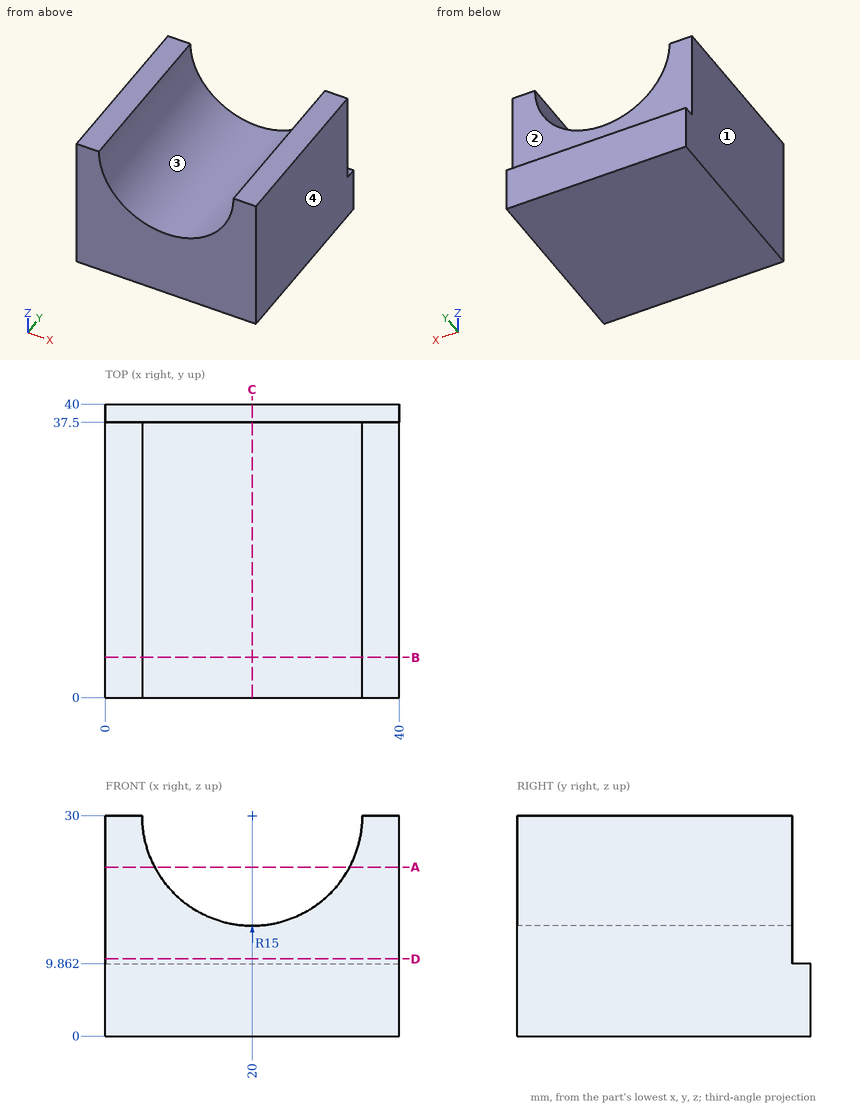
Can you work these out from the drawing? Everything is in mm from the part's minimum corner. Give positions to 0.01 mm unless a question says otherwise; leave off trailing zeros. Order: outer loops, then holes, each group sorted by start corner. A loop starts at its lowest first (then second) coordinate and runs counter-clockwise, first axis right, second up. Notation, with made-up numbers: M -38,-1 L 21,-1 A27 ccw 21,22 Z; hole C 37.25,-9.75 d11. An arc over 180 degrees is marked long. Use a Markdown table: item, result. Add a question column.
Item 1: Suppose I cut it at A-A (z = 23). List the corners of the cut face in (x, y) for me.
Item 2: Suppose I cut it at D-D (z = 10.5). List the corners of the cut face in (x, y) for me.
Item 3: Suppose I cut it at C-C (x = 20). List the corners of the cut face in (y, z) for me, then the cut area to 3 significant figures.
Item 4: We'd pull the mould along X, two halves only. Please class the marked faces 1, 2, 3 and 4: +X half, -X half, draft (parallel to the pull), parting line (faces both ways), or undercut.
Item 5: Will these pins go through, and if not, where does the flat tip stop? pin 1 (16 mm diameter, centred on x = 25.5, z = 20.5, fed in from +Y); pin 2 (1 mm diameter, centred on x = 32.5, y = 13, fed in from +Z) (1 decimal); pin 3 (4 mm diameter, centred on x = 22.5, y = 6, fed in from +Z).
Item 6: If I drill on L1, parallel to Y at x = 31.5, z = 12.5; L2, parallel to X at y = 3, z = 20; L3, parallel to Z at x = 20.5, y = 13.5, over which ranges is the centre line in solid material (lowest first)? Write a range as [from, to].
Item 7: Suppose I cut it at B-B (y = 5.5). List the corners of the cut face in (x, z) for me.
Answer sheet:
| question | item | result |
|---|---|---|
| 1 | outline | M 0,0 L 6.73,0 L 6.73,37.5 L 0,37.5 Z; M 33.27,0 L 40,0 L 40,37.5 L 33.27,37.5 Z |
| 2 | outline | M 0,0 L 40,0 L 40,37.5 L 0,37.5 Z |
| 3 | outline | M 0,0 L 40,0 L 40,9.86 L 37.5,9.86 L 37.5,15 L 0,15 Z |
| 3 | area | 587 mm² |
| 4 | face 1 | -X half |
| 4 | face 2 | draft |
| 4 | face 3 | undercut |
| 4 | face 4 | +X half |
| 5 | pin 1 | stops at y = 37.5 |
| 5 | pin 2 | stops at z = 22.5 |
| 5 | pin 3 | stops at z = 15.69 |
| 6 | L1 | y = [0, 37.5] |
| 6 | L2 | x = [0, 8.82], [31.18, 40] |
| 6 | L3 | z = [0, 15.01] |
| 7 | outline | M 0,0 L 40,0 L 40,30 L 35,30 A15 cw 5,30 L 0,30 Z |
